Part model, mm, in its own coordinate system. Face numbers are marked on the shaded views. Give positions to 0.01 mm unless a question says otherwise; leave off trailing zeros. Order: outer loops, then holes, each group sorted by start corner. A loop starts at its lowest first (then second) coordinate and runs counter-clockwise, first axis right, second up. Notation, with made-up numbers: (-17.5, 70.5) - (2.5, 70.5) arc R21 cw to (2.5, 91.5) - close; hole circle Ø11 at (-36.75, -3). An arc over 180 degrees is marked (long way). Use one line per item in the form item = value. Start each with the question number.
1. Band-saw the part on B-B, the plane z = 2.1. List the corners of the cut face in (x, y), plus the area to 3 significant figures.
2. Band-saw the part on A-A, the plane x = 0. List the corners of the cut face in (y, z).
3. Pull direction Y, two halves, no side cores. Call the marked faces 1, 2 and 3: +Y half, -Y half, draft (parallel to the pull), parting line (faces both ways), or undercut.
4. Pin check, flat tips, straight feed: P1, Ø2, axis at y = -14, z = 1, coming from the -X side; P2, Ø1.5, axis at y = 16, z = 1.5, coming from the -X side; P3, Ø2, axis at y = -3, z = 1, coming from the +X side. Stop position of each tip, or through.
5. Drill centre lines: line 1 (Y direction, x = -6.5, z = 3.55); line 2 (Y direction, x = -26, z = 3.8); line 3 (X direction, y = 17, z = 3.65). Where is each one in solid material? Low to high.
6. Band-saw the part on C-C, the plane y = 17. State how many separate pieces and enclosed holes the cut face has, plus the area to 3 significant figures.
from build123d import *

# Parameters (mm, degrees)
F0_R     = 40
F1_DEPTH = 5
F2_SIZE  = 1.5
F3_R     = 38.5
F3_R_2   = 34
F4_DEPTH = 1.5
F6_D     = 6
F6_DEPTH = 10


with BuildPart() as f1:
    # F0 (on Top) → F1 (new body)
    with BuildSketch(Plane.XY):
        Circle(F0_R)
    extrude(amount=F1_DEPTH)

    # F2
    f2_edges = [f1.edges().sort_by_distance(p)[0] for p in [
        (-40, 0, 5),
    ]]
    chamfer(f2_edges, length=F2_SIZE)

    # F3 (on face) → F4 (cut)
    with BuildSketch(Plane.XY.offset(5)):
        Circle(F3_R)
        Circle(F3_R_2, mode=Mode.SUBTRACT)
    extrude(amount=-F4_DEPTH, mode=Mode.SUBTRACT)

    # F6
    with Locations(Plane.XY.offset(5)):
        with Locations((29.444864, 17), (0, -34), (-29.444864, 17)):
            Hole(F6_D / 2, depth=F6_DEPTH)


solid = f1.part
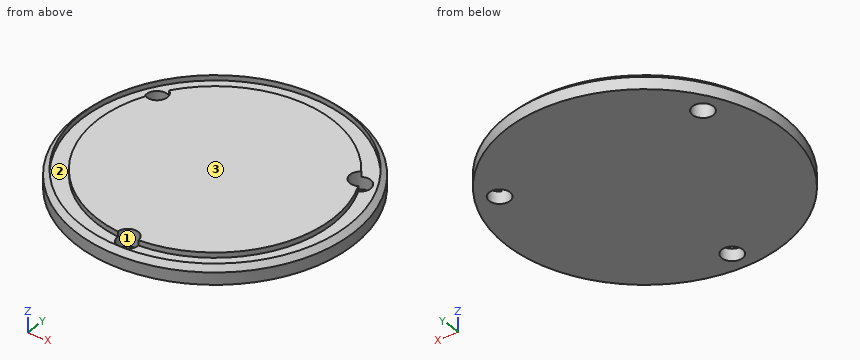
From the geometry:
q1.outline = circle Ø80 at (0, 0); hole circle Ø6 at (-29.44, 17); hole circle Ø6 at (0, -34); hole circle Ø6 at (29.44, 17)
q1.area = 4,940 mm²
q2.outline = (-40, 0) - (-37, 0) - (-37, 3.5) - (-38.5, 3.5) - (-38.5, 5) - (-40, 3.5) - close; (-31, 0) - (40, 0) - (40, 3.5) - (38.5, 5) - (38.5, 3.5) - (34, 3.5) - (34, 5) - (-31, 5) - close
q3.face_1 = undercut
q3.face_2 = undercut
q3.face_3 = draft
q4.P1 = -37.83
q4.P2 = -36.98
q4.P3 = 39.95
q5.line_1 = -39.42 to -37.95, -33.37 to 33.37, 37.95 to 39.42
q5.line_2 = -30 to -28.39, -21.91 to 21.91, 28.39 to 30
q5.line_3 = -36.04 to -34.54, -26.44 to 26.44, 34.54 to 36.04
q6.separate_pieces = 3
q6.enclosed_holes = 0
q6.area = 293 mm²
